Part model, mm, in its own coordinate system. A direction names the side the tool comes from. Give positions to 0.01 mm unless a question says otherwise; leave off trailing zeros. Order: outer loops, then holes, each group sorted by start corner. A loop starts at its lowest first (then second) coordinate and runs counter-clockwise, first axis right, second up. Notation, with made-up numbers: M 71.5,71.5 L 110.5,71.5 A6 ccw 110.5,75.5 Z; hole C -13.75,23.25 d9. An arc over 180 degrees is marked long. Write each question's results on one line, items separated by ' | '. Start each with the question number.
Autodesk Inventor part; units mm, degrees
ref_plane "YZ Plane" through (0, 0, 0) normal (1, 0, 0) x (0, 1, 0)
ref_plane "XZ Plane" through (0, 0, 0) normal (0, 1, 0) x (-1, 0, 0)
ref_plane "XY Plane" through (0, 0, 0) normal (0, 0, 1) x (1, 0, 0)
sketch "Sketch2" plane through (0, 0, 0) normal (0, 0, 1) x (1, 0, 0)
  line L0 (33, -33) -> (-33, -33)
  line L1 (-33, -33) -> (-33, 33)
  line L2 (-33, 33) -> (33, 33)
  line L3 (33, 33) -> (33, -33)
  line L4 (0, 0) -> (0, 20.7499)
  line L5 (0, 0) -> (18.2964, 0)
  point P0 (0, 33)
  point P1 (33, 0)
  dimension "d17" = 66
  dimension "d18" = 66
extrude "Extrusion1" add sketch "Sketch2" along normal blind 17
sketch "Sketch3" plane through (0, 0, 0) normal (0, 0, -1) x (-1, 0, 0)
  line L0 (33, -33) -> (33, 33)
  line L1 (33, 33) -> (-33, 33)
  line L2 (-33, 33) -> (-33, -33)
  line L3 (20, 32) -> (-20, 32)
  line L4 (-20, 32) -> (-20, 33)
  line L5 (-20, 33) -> (20, 33)
  line L6 (20, 33) -> (20, 32)
  line L7 (-20, 32) -> (-33, 32)
  line L8 (20, 32) -> (33, 32)
  point P0 (0, 0)
  point P1 (0, 33)
  dimension "d21" = 40
  dimension "d22" = 1
extrude "Extrusion2" cut sketch "Sketch3" against normal through all contours L8 L6 L1 L0 | L7 L2 L1 L4
chamfer "Chamfer1" distance 7 angle 45 2 edges at (33, 32, 8.5) (-33, 32, 8.5)
sketch "Sketch4" plane through (0, 0, 0) normal (0, 0, -1) x (-1, 0, 0)
  line L0 (-33, 25) -> (-33, -33)
  line L1 (33, -33) -> (33, 25)
  line L2 (33, 25) -> (26, 25)
  line L3 (26, 25) -> (26, 22)
  line L4 (26, 22) -> (33, 22)
  line L5 (-33, 25) -> (-26, 25)
  line L6 (-26, 25) -> (-26, 22)
  line L7 (-26, 22) -> (-33, 22)
  point P0 (0, 0)
  dimension "d28" = 7
  dimension "d29" = 3
  dimension "d30" = 7
  dimension "d31" = 3
extrude "Extrusion3" cut sketch "Sketch4" against normal through all
fillet "Fillet1" radius 1 2 edges at (-33, 25, 8.5) (33, 25, 8.5)
fillet "Fillet2" radius 3 2 edges at (33, 22, 8.5) (-33, 22, 8.5)
sketch "Sketch5" plane through (0, 0, 0) normal (0, 0, -1) x (-1, 0, 0)
  line L0 (-33, -33) -> (33, -33)
  line L1 (7.5, -33) -> (-7.5, -33)
  line L2 (-7.5, -33) -> (-7.5, -25)
  line L3 (-7.5, -25) -> (7.5, -25)
  line L4 (7.5, -25) -> (7.5, -33)
  point P0 (0, 0)
  point P1 (0, -33)
  dimension "d36" = 15
  dimension "d37" = 8
extrude "Extrusion4" cut sketch "Sketch5" against normal through all
sketch "Sketch6" plane through (0, 0, 0) normal (0, 0, -1) x (-1, 0, 0)
  line L0 (33, -33) -> (33, 19)
  line L1 (20, 33) -> (-20, 33)
  circle A0 centre (0, 7) radius 9.5
  point P0 (0, 0)
  dimension "d40" = 19
  dimension "d41" = 26
  dimension "d42" = 33
extrude "Extrusion5" cut sketch "Sketch6" against normal through all
properties part number "Holder" material "Steel, Carbon"
(1) Tool access for faces 5 (the flat face through (-28, 25, 8)), 6 (the flat face through (28, 22, 8)), 7 (the flat face through (7.5, -29, 8)): list every direction of +Z, -Z, +X, -X, +Y, -Y with a clear straight run to the whole face (end or side of a thin tool).
(2) Saw through at A-A on z = 13.25. Give the cut face in (x, y).
(3) Saw through at D-D on y = 24. Give the cut face in (x, z).
(4) Drop flat-ended pins along their axis: P1, Ø5, axis at x = 23, z = 5, coming from the +Y side; P2, Ø1, axis at y = 22, z = 8, coming from the -X side; P3, Ø4.5, axis at x = -1.5, z = 5.5, coming from the -Y side. Give the stop position or say it passes through.
(5) Probe L1, parallel to Y at x = 0, z = 4; L2, parallel to X at y = -27.5, z = 6; L3, parallel to Y at x = 2, z = 8. List the from-to ranges inside material, lowest first.
(6) Pull direction Y, two halves, no side cores. Call faces 1 (the cylindrical face through (-32.1, 21.14, 8.62)), 2 (the flat face through (20, -33, 8)), 3 (the flat face through (-23, 32, 8)), 4 (the flat face through (-33, -7, 8)): +Y half, -Y half, draft (parallel to the pull), parting line (faces both ways), or undercut.
(7) Saw through at C-C on y = 7. Give the cut face in (x, z).
(8) Saw through at B-B on x = 28. Give the cut face in (y, z), plus the area to 3 significant figures.
Taken from the geometry:
1) face 5: +Z, -Z, -X | face 6: +Z, -Z, +X | face 7: +Z, -Z, -Y
2) outline: M -33,-33 L -7.5,-33 L -7.5,-25 L 7.5,-25 L 7.5,-33 L 33,-33 L 33,19 A3 ccw 30,22 L 26,22 L 26,25 L 30.59,25 A1 ccw 31.29,26.71 L 26,32 L 20,32 L 20,33 L -20,33 L -20,32 L -26,32 L -31.29,26.71 A1 ccw -30.59,25 L -26,25 L -26,22 L -30,22 A3 ccw -33,19 Z; hole C 0,7 d19
3) outline: M -26,0 L 26,0 L 26,17 L -26,17 Z
4) P1: stops at y = 32 | P2: stops at x = -31.66 | P3: stops at y = -25
5) L1: y = -25 to -2.5, 16.5 to 33 | L2: x = -33 to -7.5, 7.5 to 33 | L3: y = -25 to -2.29, 16.29 to 33
6) face 1: undercut | face 2: -Y half | face 3: +Y half | face 4: draft
7) outline: M -33,0 L -9.5,0 L -9.5,17 L -33,17 Z; M 9.5,0 L 33,0 L 33,17 L 9.5,17 Z
8) outline: M -33,0 L 22,0 L 22,17 L -33,17 Z; M 25,0 L 30,0 L 30,17 L 25,17 Z | area: 1,020 mm²
